The listing builds one solid part. Answer for the finished solid, in the listing's coordinates (mm). Face numbers are marked on the shaded views. Give positions to 0.01 mm unless a question says otherwise; leave off trailing zeros. Loops run counter-clockwise (first coordinate to the right, second up) from the corner with the lowest first, then second, coordinate; pieces in that order, holes last.
Item 1: Section A-A, the plane z = 6 is taken. Give the vertices of the cut face in (x, y), and give its area (3 significant figures).
Item 2: Section C-C, the plane x = 148 is taken. Give the number of separate pieces and of enclosed holes in the cut face, and give its area (3 significant figures).
Item 3: The mould has two halves that part along X. Classify the marked faces 1, 2, 3 and 4: pulls with the +X half, pulls with the -X half, needs draft (parallel to the pull), parting line crosses it, or undercut.
Item 4: Section D-D, the plane y = 57.5 is taken. Give the vertices of the cut face in (x, z).
Item 5: Section B-B, the plane y = 86.5 is taken. Give the vertices of the cut face in (x, z), and give its area (3 significant figures).
Item 6: Each of these flat-tipped pins is pushed along its axis until it touches: pin 1 Ø1.5 at (x, y) = (217.5, 166) entering from -Z; pin 2 Ø4.5 at (x, y) = (110.5, 108) entering from +Z; pin 3 Ø19 at (x, y) = (146.72, 160.53) entering from -Z; pin 4 Ø6 at (y, z) = (161, 7) entering from -X. Where does it stop, or does it pass through?
Item 7: Consider line 1 along X through (y, z) = (124.5, 8); line 2 along X through (y, z) = (127, 9.25); line 3 along Y through (x, z) = (223.5, 7.25). Determine where each line is inside the solid, lowest interval first.
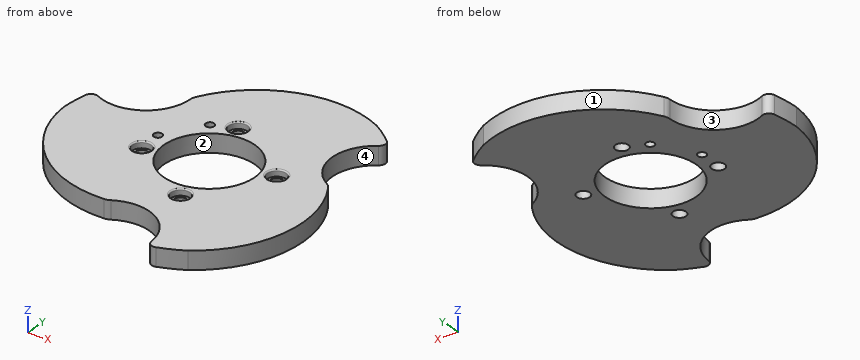
from build123d import *

# Parameters (mm, degrees)
SKETCH4_R             = 3.25
SKETCH4_R_2           = 5
SKETCH4_R_3           = 35
BOSS_EXTRUDE2_DEPTH   = 14
ESBO_O3_R             = 7.25
CORTE_EXTRUS_O1_DEPTH = 5
FILETE2_R             = 1


with BuildPart() as part:
    # Sketch4 → Boss-Extrude2 (new body)
    with BuildSketch(Plane.XY):
        with BuildLine():
            ThreePointArc((135.711956254, 40.012906067), (133.498311811, 39.078606258), (131.125704093, 38.699303642))
            ThreePointArc((131.125704093, 38.699303642), (71.046587381, 60.439214017), (43.082934706, 117.886216524))
            ThreePointArc((43.082934706, 117.886216524), (43.723303204, 128.09951793), (45.279720546, 138.213822774))
            ThreePointArc((45.279720546, 138.213822774), (47.980485983, 141.720753121), (52.406835354, 141.709543754))
            ThreePointArc((52.406835354, 141.709543754), (85.380644245, 143.225752695), (101.518008582, 172.020829263))
            ThreePointArc((101.518008582, 172.020829263), (101.815703435, 174.405051491), (102.673521593, 176.649441355))
            ThreePointArc((102.673521593, 176.649441355), (151.540394609, 217.809527477), (215.272784489, 213.303259824))
            ThreePointArc((215.272784489, 213.303259824), (223.797578714, 207.642033733), (231.77861498, 201.236984354))
            ThreePointArc((231.77861498, 201.236984354), (233.465323031, 197.144587703), (231.242440749, 193.316861385))
            ThreePointArc((231.242440749, 193.316861385), (216.068611764, 164.002600755), (232.937197408, 135.629695005))
            ThreePointArc((232.937197408, 135.629695005), (234.853146998, 134.179772586), (236.367936558, 132.314685337))
            ThreePointArc((236.367936558, 132.314685337), (247.580180254, 69.414688841), (211.811443049, 16.473953987))
            ThreePointArc((211.811443049, 16.473953987), (202.646280326, 11.921878672), (193.108826719, 8.212623207))
            ThreePointArc((193.108826719, 8.212623207), (188.72135323, 8.798089511), (186.517886141, 12.637025196))
            ThreePointArc((186.517886141, 12.637025196), (168.717906235, 40.435076885), (135.711956254, 40.012906067))
        make_face()
        with Locations((111.625067893, 123.588087508)):
            Circle(SKETCH4_R, mode=Mode.SUBTRACT)
        with Locations((146.721161104, 160.531263969)):
            Circle(SKETCH4_R_2, mode=Mode.SUBTRACT)
        with Locations((112.146853607, 105.588087508)):
            Circle(SKETCH4_R_2, mode=Mode.SUBTRACT)
        with Locations((166.723613726, 71.244356255)):
            Circle(SKETCH4_R_2, mode=Mode.SUBTRACT)
        with Locations((130.273826669, 153.217907011)):
            Circle(SKETCH4_R, mode=Mode.SUBTRACT)
        with Locations((201.365841272, 125.889036422)):
            Circle(SKETCH4_R_2, mode=Mode.SUBTRACT)
        with Locations((156.722387415, 115.887810112)):
            Circle(SKETCH4_R_3, mode=Mode.SUBTRACT)
    extrude(amount=BOSS_EXTRUDE2_DEPTH)

    # Esboço3 → Corte-extrusão1 (cut)
    with BuildSketch(Plane.XY.offset(14)):
        with Locations((201.365841272, 125.889036422)):
            Circle(ESBO_O3_R)
        with Locations((146.721161104, 160.531263969)):
            Circle(ESBO_O3_R)
        with Locations((112.146853607, 105.588087508)):
            Circle(ESBO_O3_R)
        with Locations((166.723613726, 71.244356255)):
            Circle(ESBO_O3_R)
    extrude(amount=-CORTE_EXTRUS_O1_DEPTH, mode=Mode.SUBTRACT)

    # Filete2
    filete2_edges = [part.edges().sort_by_distance(p)[0] for p in [
        (194.115841272, 125.889036422, 14),
        (139.471161104, 160.531263969, 14),
        (104.896853607, 105.588087508, 14),
        (159.473613726, 71.244356255, 14),
    ]]
    fillet(filete2_edges, radius=FILETE2_R)


solid = part.part
Worked answers:
1. outline: (43.08, 117.89) arc R85 ccw to (131.13, 38.7) arc R10 ccw to (135.71, 40.01) arc R33.99 cw to (186.52, 12.64) arc R5 ccw to (193.11, 8.21) arc R113.66 ccw to (211.81, 16.47) arc R85 ccw to (236.37, 132.31) arc R10 ccw to (232.94, 135.63) arc R33.99 cw to (231.24, 193.32) arc R5 ccw to (231.78, 201.24) arc R113.66 ccw to (215.27, 213.3) arc R85 ccw to (102.67, 176.65) arc R10 ccw to (101.52, 172.02) arc R33.99 cw to (52.41, 141.71) arc R5 ccw to (45.28, 138.21) arc R113.66 ccw to start; hole circle Ø10 at (112.15, 105.59); hole circle Ø6.5 at (111.63, 123.59); hole circle Ø70 at (156.72, 115.89); hole circle Ø6.5 at (130.27, 153.22); hole circle Ø10 at (146.72, 160.53); hole circle Ø10 at (166.72, 71.24); hole circle Ø10 at (201.37, 125.89)
1. area: 24,400 mm2
2. separate pieces: 3
2. enclosed holes: 0
2. area: 1,310 mm2
3. face 1: parting line crosses it
3. face 2: undercut
3. face 3: undercut
3. face 4: pulls with the +X half
4. outline: (74.5, 0) - (244.13, 0) - (244.13, 14) - (74.5, 14) - close
5. outline: (51.43, 0) - (137.71, 0) - (137.71, 14) - (51.43, 14) - close; (175.73, 0) - (249.43, 0) - (249.43, 14) - (175.73, 14) - close
5. area: 2,240 mm2
6. pin 1: passes through
6. pin 2: stops at z = 9
6. pin 3: stops at z = 0
6. pin 4: stops at x = 98.43
7. line 1: x = 43.39 to 108.51, 114.74 to 122.8, 190.65 to 196.56, 206.17 to 240.73
7. line 2: x = 43.61 to 123.53, 189.91 to 194.2, 208.53 to 239.45
7. line 3: y = 25.92 to 143.77, 186.23 to 207.86
